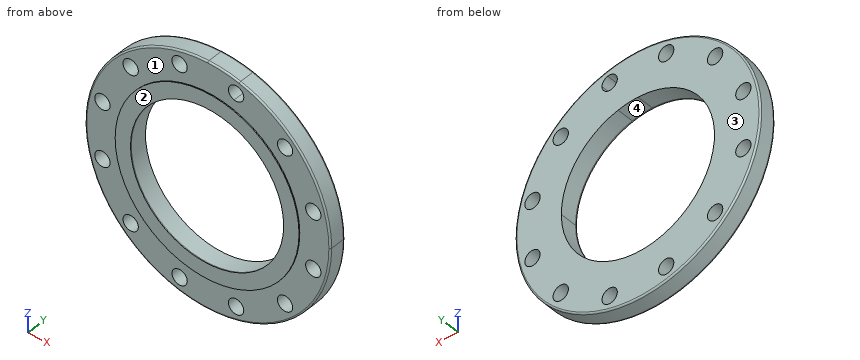
```python
from build123d import *

# Parameters (mm, degrees)
F0_R     = 12.7
F1_DEPTH = 28.448
F2_R     = 2.54
F3_R     = 152.4
F3_R_2   = 127
F4_DEPTH = 1.524


with BuildPart() as f1:
    # F0 (on Front) → F1 (new body)
    with BuildSketch(Plane.XZ):
        with BuildLine():
            ThreePointArc((0, 203.2), (-143.684098, -143.684098), (203.2, 0))
            ThreePointArc((203.2, 0), (161.209399, 123.700322), (52.59203, 196.276128))
            Line((52.59203, 196.276128), (50.126779, 187.075684))
            ThreePointArc((50.126779, 187.075684), (56.915364, 182.539697), (59.539777, 174.808426))
            ThreePointArc((59.539777, 174.808426), (54.571047, 164.732839), (43.552775, 162.541168))
            Line((43.552775, 162.541168), (32.870019, 122.67258))
            ThreePointArc((32.870019, 122.67258), (100.755874, 77.312701), (127, 0))
            ThreePointArc((127, 0), (-89.802561, -89.802561), (0, 127))
            Line((0, 127), (0, 203.2))
        make_face()
        with Locations((-127.96865, -127.96865)):
            Circle(F0_R, mode=Mode.SUBTRACT)
        with Locations((-46.839777, -174.808426)):
            Circle(F0_R, mode=Mode.SUBTRACT)
        with Locations((-174.808426, -46.839777)):
            Circle(F0_R, mode=Mode.SUBTRACT)
        with Locations((46.839777, -174.808426)):
            Circle(F0_R, mode=Mode.SUBTRACT)
        with Locations((127.96865, -127.96865)):
            Circle(F0_R, mode=Mode.SUBTRACT)
        with Locations((174.808426, -46.839777)):
            Circle(F0_R, mode=Mode.SUBTRACT)
        with Locations((-174.808426, 46.839777)):
            Circle(F0_R, mode=Mode.SUBTRACT)
        with Locations((-127.96865, 127.96865)):
            Circle(F0_R, mode=Mode.SUBTRACT)
        with Locations((-46.839777, 174.808426)):
            Circle(F0_R, mode=Mode.SUBTRACT)
        with Locations((174.808426, 46.839777)):
            Circle(F0_R, mode=Mode.SUBTRACT)
        with Locations((127.96865, 127.96865)):
            Circle(F0_R, mode=Mode.SUBTRACT)
        with BuildLine():
            Line((50.126779, 187.075684), (52.59203, 196.276128))
            ThreePointArc((52.59203, 196.276128), (26.522922, 201.461596), (0, 203.2))
            Line((0, 203.2), (0, 127))
            ThreePointArc((0, 127), (16.576826, 125.913497), (32.870019, 122.67258))
            Line((32.870019, 122.67258), (43.552775, 162.541168))
            ThreePointArc((43.552775, 162.541168), (34.572519, 178.095428), (50.126779, 187.075684))
        make_face()
    extrude(amount=F1_DEPTH)

    # F2
    f2_edges = [f1.edges().sort_by_distance(p)[0] for p in [
        (-203.2, -28.448, 0),
        (-203.2, 0, 0),
    ]]
    fillet(f2_edges, radius=F2_R)

    # F3 (on face) → F4 (join)
    with BuildSketch(Plane.XZ.offset(28.448)):
        Circle(F3_R)
        Circle(F3_R_2, mode=Mode.SUBTRACT)
    extrude(amount=F4_DEPTH)


solid = f1.part
```
Input: part model. Units: mm. Frame: model coordinates. Face numbers are marked on the shaded views. A direction names the side the tool comes from. Coordinates: 2 decimals unless noted, no trailing zeros. Use a Markdown table: item, result. Add a question column.
1) Line query: L1, parallel to X at y = -4.75, z = -45; L2, parallel to X at y = -21.5, z = -134; L3, parallel to Z at x = 0, y = -29.1. Output: solid intervals per line, ascending. Write a range as from..to.
2) Pin query (flat end, axial travel): P1, Ø4, axis at x = 100, y = -9.5, coming from the +Z side; P2, Ø1, axis at y = -11, z = 94.5, coming from the -X side; P3, Ø1.5, axis at y = -17.5, z = 112, coming from the -X side. Return the tip coordinate at first contact, or that it passes through.
3) Section A-A, the plane y = -20. Give the number of separate pieces and of enclosed holes in the cut face, plus the area to 3 significant figures.
4) Draft query along Z for the marked faces 3 and 4. Return one class per face: +Z half, -Z half, draft (parallel to the pull), parting line (faces both ways), or undercut.
5) Set-up query: the marked faces 1 and 2. Return all of +Z, -Z, +X, -X, +Y, -Y with unobstructed straight access to the full face (end or side cutting, diameter ignored); none if empty.
Answer below:
| question | item | result |
|---|---|---|
| 1 | L1 | -198.15..-187.37, -162.24..-118.76, 118.76..162.24, 187.37..198.15 |
| 1 | L2 | -152.76..-139.15, -116.79..116.79, 139.15..152.76 |
| 1 | L3 | -152.4..-127, 127..152.4 |
| 2 | P1 | z = 178.01 |
| 2 | P2 | x = -180.15 |
| 2 | P3 | x = -170.04 |
| 3 | separate pieces | 1 |
| 3 | enclosed holes | 13 |
| 3 | area | 73,000 mm2 |
| 4 | face 3 | draft |
| 4 | face 4 | undercut |
| 5 | face 1 | -Y |
| 5 | face 2 | +Z, -Z, +X, -X, -Y |
